Geometry check sheet. Reference: the model listing, model coordinates, mm. Face numbers are marked on the shaded views. A direction names the side the tool comes from. Round coordinates to 2 decimals unless told otherwise and drop trailing zeros. Loops run counter-clockwise (first coordinate to the right, second up) from the corner with the lowest first, then second, coordinate; pieces in that order, holes last. Notation, with made-up numbers: M -18,-4.75 L -8,-4.75 A16 ccw -8,5.25 Z; hole C -1,-25.5 d2. An arc over 180 degrees is marked long. Write item = value, one per line.
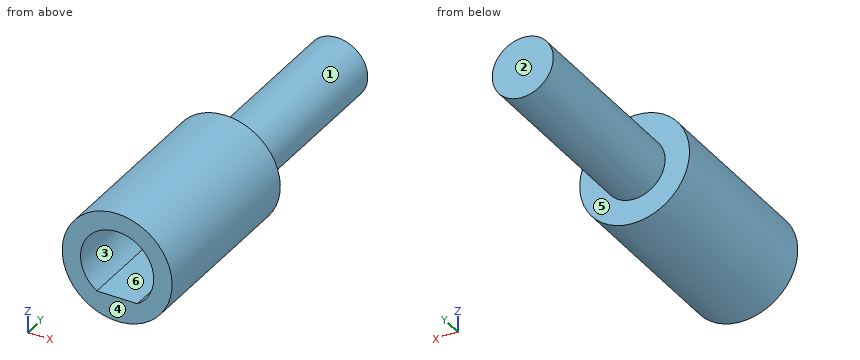
from build123d import *

# Parameters (mm, degrees)
SKETCH2_R           = 4.5
BOSS_EXTRUDE1_DEPTH = 12
SKETCH3_R           = 4.5
BOSS_EXTRUDE2_DEPTH = 3
SKETCH4_R           = 2.5
BOSS_EXTRUDE3_DEPTH = 15.5


with BuildPart() as part:
    # Sketch2 → Boss-Extrude1 (new body)
    with BuildSketch(Plane(origin=(0, 0, 0), x_dir=(1, 0, 0), z_dir=(0, 1, 0))):
        with Locations(Location((0, 0, 0), (0, 0, 270))):
            Circle(SKETCH2_R)
        with BuildLine():
            ThreePointArc((1.658312395, 2.5), (0, -3), (-1.658312395, 2.5))
            Line((-1.658312395, 2.5), (1.658312395, 2.5))
        make_face(mode=Mode.SUBTRACT)
    extrude(amount=BOSS_EXTRUDE1_DEPTH)

    # Sketch3 → Boss-Extrude2 (add)
    with BuildSketch(Plane(origin=(0, 12, 0), x_dir=(1, 0, 0), z_dir=(0, 1, 0))):
        with Locations(Location((0, 0, 0), (0, 0, 270))):
            Circle(SKETCH3_R)
    extrude(amount=BOSS_EXTRUDE2_DEPTH)

    # Sketch4 → Boss-Extrude3 (add)
    with BuildSketch(Plane(origin=(0, 15, 0), x_dir=(1, 0, 0), z_dir=(0, 1, 0))):
        with Locations(Location((0, 0, 0), (0, 0, 270))):
            Circle(SKETCH4_R)
    extrude(amount=BOSS_EXTRUDE3_DEPTH)


solid = part.part
(1) Sectioned sample at A-A on x = 0. Record the cut outline in (y, z).
Result set:
outline = M 0,-4.5 L 15,-4.5 L 15,-2.5 L 30.5,-2.5 L 30.5,2.5 L 15,2.5 L 15,4.5 L 0,4.5 L 0,3 L 12,3 L 12,-2.5 L 0,-2.5 Z
(2) Tool access check on the marked faces 4, 5 and 6. Record the directions out of +Z, -Z, +X, -X, +Y, -Y that give a thin tool (end or side, any length) a straight path to the whole face; none if there is none.
Result set:
face_4 = +Z, -Z, +X, -X, -Y
face_5 = +Y
face_6 = -Y
(3) Sectioned sample at D-D on y = 28. Record the cut outline in (x, z).
Result set:
outline = C 0,0 d5
(4) Depth check by flat-ended pin: pin 1 Ø3 at (x, y) = (2, 13.5) entering from -Z. Enter the tip coordinate at first touch or a pass-through.
Result set:
pin_1 = -4.47
(5) Release check for a two-part mould opening along Z. For the marked faces 1, 2 and 3 record: released by +Z, released by -Z, zero draft, split by the parting line, or undercut.
Result set:
face_1 = split by the parting line
face_2 = zero draft
face_3 = undercut
(6) Sectioned sample at C-C on y = 9. Record the cut outline in (x, z).
Result set:
outline = C 0,0 d9; hole M -1.66,-2.5 L 1.66,-2.5 A3 ccw long Z
(7) Sectioned sample at B-B on z = 0. Record the cut outline in (x, y), then the cut area to 4 significant figures.
Result set:
outline = M -4.5,0 L -3,0 L -3,12 L 3,12 L 3,0 L 4.5,0 L 4.5,15 L 2.5,15 L 2.5,30.5 L -2.5,30.5 L -2.5,15 L -4.5,15 Z
area = 140.5 mm2
(8) Material ranges on line 1 along X through (y, z) = (6, 0); line 2 along Y through (x, z) = (-0.25, -2.75); line 3 along Y through (x, z) = (-1.25, 0.5), recorded low to high. Write a range as from..to.
Result set:
line_1 = -4.5..-3, 3..4.5
line_2 = 0..15
line_3 = 12..30.5
